```python
from build123d import *

# Parameters (mm, degrees)
SKETCH1_R           = 15
BOSS_EXTRUDE1_DEPTH = 21
SKETCH2_W           = 21
SKETCH2_H           = 30
BOSS_EXTRUDE2_DEPTH = 25.2
SKETCH3_R           = 16
BOSS_EXTRUDE3_DEPTH = 127.2
SKETCH4_R           = 11
BOSS_EXTRUDE4_DEPTH = 2.3
SKETCH6_R           = 5
BOSS_EXTRUDE6_DEPTH = 18.7
BOSS_EXTRUDE7_DEPTH = 6
SKETCH7_R           = 1.5
CUT_EXTRUDE1_DEPTH  = 10
CIRPATTERN1_COUNT   = 6


with BuildPart() as part:
    # Sketch1 → Boss-Extrude1 (new body)
    with BuildSketch(Plane.XY):
        with Locations(Location((0, 0, 0), (0, 0, 180))):
            Circle(SKETCH1_R)
    extrude(amount=BOSS_EXTRUDE1_DEPTH)

    # Sketch2 → Boss-Extrude2 (add)
    with BuildSketch(Plane(origin=(0, 0, 0), x_dir=(0, 0, -1), z_dir=(1, 0, 0))):
        with Locations((-10.5, 0)):
            Rectangle(SKETCH2_W, SKETCH2_H)
    extrude(amount=BOSS_EXTRUDE2_DEPTH)

    # Sketch3 → Boss-Extrude3 (add)
    with BuildSketch(Plane.XY.offset(21)):
        with Locations(Location((0, 0, 0), (0, 0, 290.364134806))):
            Circle(SKETCH3_R)
    extrude(amount=BOSS_EXTRUDE3_DEPTH)

    # Sketch4 → Boss-Extrude4 (add)
    with BuildSketch(Plane.XY.offset(148.2)):
        Circle(SKETCH4_R)
    extrude(amount=BOSS_EXTRUDE4_DEPTH)

    # Sketch6 → Boss-Extrude6 (add)
    with BuildSketch(Plane.XY.offset(150.5)):
        Circle(SKETCH6_R)
    extrude(amount=BOSS_EXTRUDE6_DEPTH)

    # Sketch5 → Boss-Extrude7 (add)
    with BuildSketch(Plane(origin=(0, 0, 0), x_dir=(0, 0, -1), z_dir=(1, 0, 0))):
        with BuildLine():
            Line((-155.7, 1.5), (-164.7, 1.5))
            ThreePointArc((-164.7, 1.5), (-166.2, 0), (-164.7, -1.5))
            Line((-164.7, -1.5), (-155.7, -1.5))
            ThreePointArc((-155.7, -1.5), (-154.2, 0), (-155.7, 1.5))
        make_face()
    extrude(amount=-BOSS_EXTRUDE7_DEPTH)

    # Sketch7 → Cut-Extrude1 (cut)
    with BuildSketch(Plane.XY.offset(148.2)):
        with Locations((13.5, 0)):
            Circle(SKETCH7_R)
    cut_extrude1 = extrude(amount=-CUT_EXTRUDE1_DEPTH, mode=Mode.SUBTRACT)

    # CirPattern1: Cut-Extrude1 ×6 about axis
    cirpattern1_axis = Axis((0, 0, 0), (0, 0, 1))
    for i in range(1, CIRPATTERN1_COUNT):
        add(cut_extrude1.rotate(cirpattern1_axis, i * 360 / CIRPATTERN1_COUNT), mode=Mode.SUBTRACT)


solid = part.part
```
Read the model definition and answer for the solid it produces. Units are mm, in the model's axes. A direction names the side the tool comes from. Give positions to 0.01 mm unless a question says otherwise; leave off trailing zeros. Write each loop counter-clockwise with the first axis right and the second up, starting at its lowest first coordinate (ties: lowest second). Pieces come first, ordered by that corner, then holes. Notation, with made-up numbers: (-5.75, 63.5) -> (12.25, 63.5) arc R26 cw to (12.25, 84.5) -> close; hole circle Ø4 at (77, 74.5). An arc over 180 degrees is marked (long way). Answer in a Markdown table with one row per item.
1) Determine the mould class of faces 6 (the flat face through (12, 15, 11)), 7 (the cylindrical face through (4.77, 1.5, 159.72)), 8 (the cylindrical face through (-7.856, 12.705, 143.27)) for opening direction X: released by +X, released by -X, zero draft, split by the parting line, or undercut.
Results list:
| item | result |
|---|---|
| face 6 | zero draft |
| face 7 | split by the parting line |
| face 8 | undercut |
2) A tool of negligible diameter and unlimited length cuts with its end or side. For faces 1 (the flat face through (-7, 12, 138.2)), 2 (the flat face through (0, 0, 169.2)), 3 (the flat face through (12, -15, 11)), 4 (the flat face through (25.2, 0, 11)), 5 (the flat face through (-15, 3, 21)), from which of +Z, -Z, +X, -X, +Y, -Y can it reach the whole face along a straight path? Write none if from no direction.
Results list:
| item | result |
|---|---|
| face 1 | +Z |
| face 2 | +Z, +X, -X, +Y, -Y |
| face 3 | -Z, +X, -X, -Y |
| face 4 | +Z, -Z, +X, +Y, -Y |
| face 5 | -Z, -X |
3) Section B-B on x = 13.5 is taken. Give the vertices of the cut face in (y, z), plus the area to 3 significant figures.
Results list:
| item | result |
|---|---|
| outline | (-15, 0) -> (15, 0) -> (15, 21) -> (8.59, 21) -> (8.59, 148.2) -> (1.5, 148.2) -> (1.5, 138.2) -> (-1.5, 138.2) -> (-1.5, 148.2) -> (-8.59, 148.2) -> (-8.59, 21) -> (-15, 21) -> close |
| area | 2,780 mm^2 |
4) Section A-A on y = 0 is taken. Give the vertices of the cut face in (x, z), plus the area to 3 significant figures.
Results list:
| item | result |
|---|---|
| outline | (-16, 21) -> (-15, 21) -> (-15, 0) -> (25.2, 0) -> (25.2, 21) -> (16, 21) -> (16, 148.2) -> (15, 148.2) -> (15, 138.2) -> (12, 138.2) -> (12, 148.2) -> (11, 148.2) -> (11, 150.5) -> (5, 150.5) -> (5, 169.2) -> (-5, 169.2) -> (-5, 166.2) -> (-6, 166.2) -> (-6, 154.2) -> (-5, 154.2) -> (-5, 150.5) -> (-11, 150.5) -> (-11, 148.2) -> (-12, 148.2) -> (-12, 138.2) -> (-15, 138.2) -> (-15, 148.2) -> (-16, 148.2) -> close |
| area | 5,100 mm^2 |
5) Each of these flat-tipped pins is pushed along its axis until it touches: pin 1 Ø0.9 at (x, y) = (-6.5, -12) entering from +Z; pin 2 Ø3 at (y, z) = (4, 35.5) entering from -X; pin 3 Ø2.5 at (y, z) = (0.5, 158.5) entering from -X. Where does it stop, or does it pass through?
Results list:
| item | result |
|---|---|
| pin 1 | z = 138.2 |
| pin 2 | x = -15.8 |
| pin 3 | x = -6 |
6) Straight lines are drawn through the part: line 1 (Y direction, x = 6.75, z = 143); line 2 (Z direction, x = 13, y = 14); line 3 (Z direction, x = 15, y = -5). For each, find the intervals that lie inside material, in ascending order. Write a range as [from, to].
Results list:
| item | result |
|---|---|
| line 1 | [-14.51, -13.19], [-10.19, 10.19], [13.19, 14.51] |
| line 2 | [0, 21] |
| line 3 | [0, 148.2] |
7) Section C-C on z = 113 is taken. Give the vertices of the cut face in (x, y).
Results list:
| item | result |
|---|---|
| outline | circle Ø32 at (0, 0) |
